from build123d import *

# Parameters (mm, degrees)
SKETCH1_R           = 10
BOSS_EXTRUDE1_DEPTH = 170
SKETCH2_W           = 25
SKETCH2_H           = 15
BOSS_EXTRUDE3_DEPTH = 10
BOSS_EXTRUDE4_START = -10
SKETCH3_R           = 7.5
BOSS_EXTRUDE4_DEPTH = 20
SKETCH4_R           = 5
CUT_EXTRUDE1_DEPTH  = 80
SKETCH5_R           = 5
CUT_EXTRUDE2_DEPTH  = 5
BOSS_EXTRUDE5_DEPTH = 15
SKETCH7_R           = 2.5
CUT_EXTRUDE3_DEPTH  = 15


with BuildPart() as part:
    # Sketch1 → Boss-Extrude1 (new body)
    with BuildSketch(Plane(origin=(0, 0, 0), x_dir=(1, 0, 0), z_dir=(0, 1, 0))):
        with Locations(Location((0, 0, 0), (0, 0, 270))):
            Circle(SKETCH1_R)
    extrude(amount=BOSS_EXTRUDE1_DEPTH)

    # Sketch2 → Boss-Extrude3 (add, symmetric)
    with BuildSketch(Plane.XY):
        with Locations((0, 40)):
            Rectangle(SKETCH2_W, SKETCH2_H)
    extrude(amount=BOSS_EXTRUDE3_DEPTH, both=True)

    # Sketch3 → Boss-Extrude4 (add, symmetric)
    with BuildSketch(Plane.XY.offset(10).offset(BOSS_EXTRUDE4_START)):
        with Locations(Location((0, 40, 0), (0, 0, 270))):
            Circle(SKETCH3_R)
    extrude(amount=BOSS_EXTRUDE4_DEPTH, both=True)

    # Sketch4 → Cut-Extrude1 (cut)
    with BuildSketch(Plane(origin=(0, 170, 0), x_dir=(1, 0, 0), z_dir=(0, 1, 0))):
        with Locations(Location((0, 0, 0), (0, 0, 270))):
            Circle(SKETCH4_R)
    extrude(amount=-CUT_EXTRUDE1_DEPTH, mode=Mode.SUBTRACT)

    # Sketch5 → Cut-Extrude2 (cut)
    with BuildSketch(Plane(origin=(0, 0, -20), x_dir=(-1, 0, 0), z_dir=(0, 0, -1))):
        with Locations((0, 40)):
            Circle(SKETCH5_R)
    cut_extrude2 = extrude(amount=-CUT_EXTRUDE2_DEPTH, mode=Mode.SUBTRACT)

    # Mirror1: Cut-Extrude2 across plane
    add(cut_extrude2.mirror(Plane.XY), mode=Mode.SUBTRACT)

    # Sketch6 → Boss-Extrude5 (add)
    with BuildSketch(Plane.XZ.offset(-32.5)):
        with BuildLine():
            Line((-12.5, 10), (-12.5, -10))
            ThreePointArc((-12.5, -10), (-22.5, 0), (-12.5, 10))
        make_face()
    extrude(amount=-BOSS_EXTRUDE5_DEPTH)

    # Sketch7 → Cut-Extrude3 (cut)
    with BuildSketch(Plane.XZ.offset(-32.5)):
        with Locations(Location((-18, 0, 0), (0, 0, 270))):
            Circle(SKETCH7_R)
    extrude(amount=-CUT_EXTRUDE3_DEPTH, mode=Mode.SUBTRACT)


solid = part.part
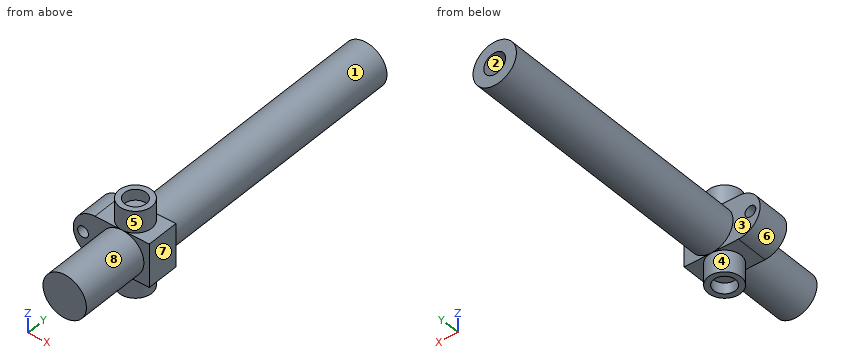
Design review of the part built by this model. Coordinates are the model's own, in mm. Face numbers are marked on the shaded views. A direction names the side the tool comes from. Coordinates: 2 decimals unless noted, no trailing zeros. Order: outer loops, then holes, each group sorted by start corner. A loop starts at its lowest first (then second) coordinate and runs counter-clockwise, first axis right, second up. Notation, with made-up numbers: (64, -31.5) -> (106, -31.5) arc R13 cw to (106, -9.5) -> close; hole circle Ø11 at (-8, -2). An arc over 180 degrees is marked (long way). One line per item, written item: value.
1) We need section B-B, the plane y = 40. Give the boundary of the cut face in (x, z).
Output values:
outline: (-12.5, -10) -> (-7.5, -10) -> (-7.5, -20) -> (-5, -20) -> (-5, -15) -> (5, -15) -> (5, -20) -> (7.5, -20) -> (7.5, -10) -> (12.5, -10) -> (12.5, 10) -> (7.5, 10) -> (7.5, 20) -> (5, 20) -> (5, 15) -> (-5, 15) -> (-5, 20) -> (-7.5, 20) -> (-7.5, 10) -> (-12.5, 10) arc R10 ccw to start; hole circle Ø5 at (-18, 0)
2) Clearance check with flat-ended pins moving along their axes: P1, Ø9, axis at x = 0, y = 40, coming from the -Z side; P2, Ø5, axis at x = -2, y = 85, coming from the +Z side; P3, Ø5, axis at x = -17.5, z = 5.5, coming from the +Y side; P4, Ø3, axis at x = -18, z = 0, coming from the +Y side. State where each tip first meets the part, or that it passes through.
Output values:
P1: stops at z = -15
P2: stops at z = 10
P3: stops at y = 47.5
P4: passes through
3) We need section C-C, the plane z = -6.5. Give the boundary of the cut face in (x, y), then the cut area to 3 significant figures.
Output values:
outline: (-20.1, 32.5) -> (-7.6, 32.5) -> (-7.6, 0) -> (7.6, 0) -> (7.6, 32.5) -> (12.5, 32.5) -> (12.5, 47.5) -> (7.6, 47.5) -> (7.6, 170) -> (-7.6, 170) -> (-7.6, 47.5) -> (-20.1, 47.5) -> close
area: 2,840 mm2
4) We need section A-A, the plane z = 0. Give the boundary of the cut face in (x, y), then the cut area to 3 significant figures.
Output values:
outline: (-22.5, 32.5) -> (-20.5, 32.5) -> (-20.5, 47.5) -> (-22.5, 47.5) -> close; (-15.5, 32.5) -> (-10, 32.5) -> (-10, 0) -> (10, 0) -> (10, 32.5) -> (12.5, 32.5) -> (12.5, 47.5) -> (10, 47.5) -> (10, 170) -> (5, 170) -> (5, 90) -> (-5, 90) -> (-5, 170) -> (-10, 170) -> (-10, 47.5) -> (-15.5, 47.5) -> close
area: 2,750 mm2
5) We need section D-D, the plane y = 70. Give the boundary of the cut face in (x, z), then the cut area to 3 significant figures.
Output values:
outline: circle Ø20 at (0, 0)
area: 314 mm2
6) To check wall thickness, follow probe 1 along X at (y, z) = (41.75, 0); probe 2 along Y at (x, z) = (0, 18.4); probe 3 along Z at (x, y) = (-2, 125). State the ranges of each line that lie inside material, in increasing order. Write a range as [from, to].
Output values:
probe 1: x = [-22.5, -20.5], [-15.5, 12.5]
probe 2: y = [32.5, 35], [45, 47.5]
probe 3: z = [-9.8, -4.58], [4.58, 9.8]
7) Draft analysis for pull direction X (two halves, no side actions). For the marked faces 1, 2 and 3, state which applies: +X half, -X half, draft (parallel to the pull), parting line (faces both ways), or undercut.
Output values:
face 1: parting line
face 2: undercut
face 3: draft
8) Machinability: for the marked faces 4, 5, 6, 7 and 8, which of the approach directions +Z, -Z, +X, -X, +Y, -Y give a long, thin tool a straight path to every point of the face, cutting with its end or side? Answer none if there is none.
Output values:
face 4: -Z
face 5: +Z
face 6: -X, +Y, -Y
face 7: +Z, -Z, +X, +Y, -Y
face 8: -Y
